The listing builds one solid part. Answer for the finished solid, in the listing's coordinates (mm). A direction names the side the tool comes from. Round coordinates to 2 decimals unless told otherwise and drop trailing zeros. Write each loop counter-clockwise with the first axis right and the second up, starting at its lowest first coordinate (ties: lowest second). Pieces come first, ordered by that corner, then holes. Notation, with made-up numbers: (85, -14) - (116, -14) arc R9 ccw to (116, -6) - close; hole circle Ø1 at (29.5, -4.5). An arc over 180 degrees is marked (long way). Use a Markdown table: item, result. Add a question column.
1) A tool of negligible diameter and unlimited length cuts with its end or side. For faces 1 (the flat face through (16.72, 7.92, 2.54)), 2 (the flat face through (-15.22, 10.52, 2.54)), 3 (the flat face through (1.5, -19, 3)), 4 (the flat face through (15.27, 10.55, 2.54)), 5 (the cylindrical face through (-15.23, 2.95, 1.48)), from which of +Z, -Z, +X, -X, +Y, -Y can it reach the whole face along a straight path? Write none if from no direction.
2) A cutting plane is placed at A-A (x = 0). Give the vertices of the cut face in (y, z).
3) A cutting plane is placed at C-C (y = -16). Give the vertices of the cut face in (x, z), then the cut area to 3 significant figures.
4) Find the intervals of material crossed by probe 1 along Y at (x, z) = (0, 0.85); probe 2 along X at (y, z) = (0, 1.05); probe 3 along Y at (x, z) = (0, 2.3), in increasing order. Write a range as from..to.
5) A cutting plane is placed at B-B (z = 4.4). State how many separate pieces and enclosed holes the cut face has, then the cut area to 3 significant figures.
6) Each of these flat-tipped pins is pushed along its axis until it touches: P1, Ø2.5, axis at x = -14.29, y = -8.25, coming from the -Z side; P2, Ø1.2, axis at y = -19, z = 1.5, coming from the -X side; P3, Ø1.5, axis at x = -7, z = 1.5, coming from the -Y side; P4, Ø3, axis at x = -17, y = 7, coming from the -Z side. Where does it stop, or does it pass through?
```python
from build123d import *

# Parameters (mm, degrees)
SKETCH1_R          = 20.5
SKETCH1_R_2        = 13.5
SKETCH1_R_3        = 1.5875
EXTRUDE1_DEPTH     = 5
CUT_EXTRUDE1_DEPTH = 30.419381367
CIRPATTERN1_COUNT  = 3
SKETCH5_R          = 1.5
CUT_EXTRUDE2_DEPTH = 3


with BuildPart() as part:
    # Sketch1 → Extrude1 (new body)
    with BuildSketch(Plane.XY):
        Circle(SKETCH1_R)
        Circle(SKETCH1_R_2, mode=Mode.SUBTRACT)
        with Locations((0, 16.5)):
            Circle(SKETCH1_R_3, mode=Mode.SUBTRACT)
        with Locations((14.289419162, -8.25)):
            Circle(SKETCH1_R_3, mode=Mode.SUBTRACT)
        with Locations((-14.289419162, -8.25)):
            Circle(SKETCH1_R_3, mode=Mode.SUBTRACT)
    extrude(amount=EXTRUDE1_DEPTH)

    # Sketch2 → Cut-Extrude1 (cut, through all)
    with BuildSketch(Plane.XY.offset(5)):
        with BuildLine():
            ThreePointArc((1.5, -16.5), (0, -15), (-1.5, -16.5))
            Line((-1.5, -16.5), (-1.5, -20.4450483))
            ThreePointArc((-1.5, -20.4450483), (0, -20.5), (1.5, -20.4450483))
            Line((1.5, -20.4450483), (1.5, -16.5))
        make_face()
    cut_extrude1 = extrude(amount=-CUT_EXTRUDE1_DEPTH, mode=Mode.SUBTRACT)

    # Sketch4 → Cut-Revolve3 (revolve, cut)
    with BuildSketch(Plane(origin=(0, 0, 0), x_dir=(1, 0, 0), z_dir=(0, 1, 0))):
        Polygon((-13.5, -2.5), (-13.5, -1.5), (-14.5, -2.5), align=None)
        Polygon((-13.5, -3.5), (-13.5, -2.5), (-14.5, -2.5), align=None)
    revolve(axis=Axis((0, 0, 0), (0, 0, 1)), mode=Mode.SUBTRACT)

    # CirPattern1: Cut-Extrude1 ×3 about axis
    cirpattern1_axis = Axis((0, 0, 0), (0, 0, 1))
    for i in range(1, CIRPATTERN1_COUNT):
        add(cut_extrude1.rotate(cirpattern1_axis, i * 360 / CIRPATTERN1_COUNT), mode=Mode.SUBTRACT)

    # Sketch5 → Cut-Extrude2 (cut)
    with BuildSketch(Plane(origin=(0, 0, 0), x_dir=(-1, 0, 0), z_dir=(0, 0, -1))):
        with Locations((15.937776134, 4.270514244)):
            Circle(SKETCH5_R)
        with BuildLine():
            Line((12.903599864, 7.675974851), (14.551956835, 3.696489096))
            ThreePointArc((14.551956835, 3.696489096), (15.645140651, 5.741692165), (17.437776134, 4.270514244))
            ThreePointArc((17.437776134, 4.270514244), (17.106740008, 3.330554957), (16.259744852, 2.805476312))
            Line((16.259744852, 2.805476312), (20.169765215, 3.664774367))
            ThreePointArc((20.169765215, 3.664774367), (19.491013781, 6.352195037), (18.45593121, 8.923486044))
            Line((18.45593121, 8.923486044), (15.039419162, 6.950961894))
            ThreePointArc((15.039419162, 6.950961894), (13.807259964, 6.829604806), (12.903599864, 7.675974851))
        make_face()
    extrude(amount=-CUT_EXTRUDE2_DEPTH, mode=Mode.SUBTRACT)


solid = part.part
```
Entries:
| question | item | result |
|---|---|---|
| 1 | face 1 | +Z, -Z |
| 1 | face 2 | +Z, -Z, -X |
| 1 | face 3 | +Z, -Z, -Y |
| 1 | face 4 | +Z, -Z, +X |
| 1 | face 5 | -Z |
| 2 | outline | (-15, 0) - (-13.5, 0) - (-13.5, 1.5) - (-14.5, 2.5) - (-13.5, 3.5) - (-13.5, 5) - (-15, 5) - close; (13.5, 0) - (14.91, 0) - (14.91, 5) - (13.5, 5) - (13.5, 3.5) - (14.5, 2.5) - (13.5, 1.5) - close; (18.09, 0) - (20.5, 0) - (20.5, 5) - (18.09, 5) - close |
| 3 | outline | (-12.82, 0) - (-1.41, 0) - (-1.41, 5) - (-12.82, 5) - close; (1.41, 0) - (12.82, 0) - (12.82, 5) - (1.41, 5) - close |
| 3 | area | 114 mm² |
| 4 | probe 1 | y = -15..-13.5, 13.5..14.91, 18.09..20.5 |
| 4 | probe 2 | x = -20.5..-13.5, 13.5..20.5 |
| 4 | probe 3 | y = -15..-14.3, 14.3..14.91, 18.09..20.5 |
| 5 | separate pieces | 1 |
| 5 | enclosed holes | 4 |
| 5 | area | 678 mm² |
| 6 | P1 | passes through |
| 6 | P2 | stops at x = -9.04 |
| 6 | P3 | stops at y = -19.52 |
| 6 | P4 | stops at z = 3 |
